Autodesk Inventor part; units mm, degrees
ref_plane "YZ Plane" through (0, 0, 0) normal (1, 0, 0) x (0, 1, 0)
ref_plane "XZ Plane" through (0, 0, 0) normal (0, 1, 0) x (-1, 0, 0)
ref_plane "XY Plane" through (0, 0, 0) normal (0, 0, 1) x (1, 0, 0)
sketch "Sketch1" plane through (0, 0, 0) normal (0, 0, 1) x (1, 0, 0)
  circle A0 centre (0, 0) radius 374.904
  dimension "d0" = 749.808
extrude "Extrusion1" add sketch "Sketch1" along normal blind 25.4
sketch "Sketch2" plane through (0, 0, 0) normal (0, 0, 1) x (1, 0, 0)
  circle A0 centre (0, 0) radius 355.854
  dimension "d3" = 711.708
extrude "Extrusion2" add sketch "Sketch2" along normal blind 50
sketch "Sketch3" plane through (0, 0, 0) normal (0, 0, 1) x (1, 0, 0)
  circle A0 centre (0, 0) radius 349.25
  dimension "d6" = 698.5
extrude "Extrusion3" add sketch "Sketch3" along normal blind 1330.7314
sketch "Sketch4" plane through (0, 0, 1330.7314) normal (0, 0, 1) x (1, 0, 0)
  circle A0 centre (-6.35, 0) radius 317.5
  point P0 (0, 0)
  dimension "d9" = 635
  dimension "d21" = 6.35
extrude "Extrusion4" cut sketch "Sketch4" against normal through all
chamfer "Chamfer1" distance 0.7937 angle 45 1 edges at (-374.904, 0, 25.4)
fillet "Fillet1" radius 0.7937 1 edges at (-355.854, 0, 25.4)
fillet "Fillet2" radius 0.7937 1 edges at (-349.25, 0, 50)
sketch "Sketch5" plane through (0, 0, 0) normal (0, 1, 0) x (-1, 0, 0)
  line L0 (-311.15, 1330.7314) -> (323.85, 1330.7314)
  line L1 (-311.15, 1330.7314) -> (323.85, 797.9031)
  line L2 (323.85, 797.9031) -> (349.25, 797.9031)
  line L3 (349.25, 797.9031) -> (349.25, 1330.7314)
  line L4 (349.25, 1330.7314) -> (323.85, 1330.7314)
  line L5 (349.25, 50.7937) -> (349.25, 1330.7314) construction
  point P0 (0, 0)
  dimension "d18" = 40
extrude "Extrusion5" cut sketch "Sketch5" along normal through all both and the other way through all
properties part number "A1-19010-200-02 HCWI nozzle insert" material "Iron, Cast"
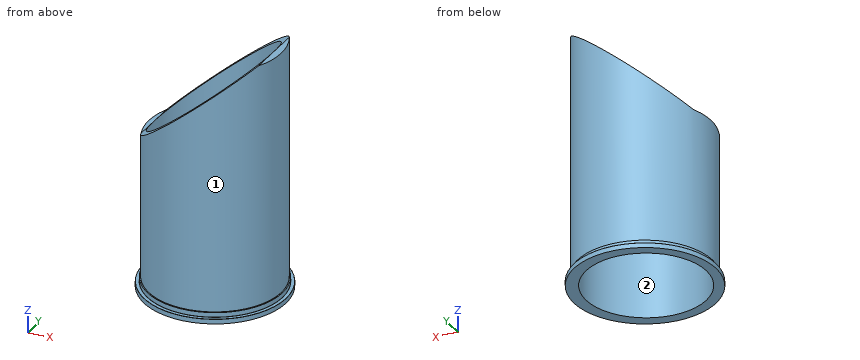
For this review, take the finished solid that the model builds, in its own axes (mm). Face numbers are marked on the shaded views. Give positions to 0.01 mm unless a question says otherwise; leave off trailing zeros. Loops run counter-clockwise (first coordinate to the right, second up) from the corner with the lowest first, then second, coordinate; pieces in that order, holes last. Notation, with made-up numbers: M 60.25,-5 L 83.25,-5 A20 cw 83.25,13 Z; hole C 64,54 d7. An arc over 180 degrees is marked long. Answer as a JSON object with one key per item and string values. Group by question number.
Q1. Add section A-A on z = 229.5. Give the boundary of the cut face in (x, y), and give its area (3 significant figures).
Q2. Add section B-B on x = 0. Give the boundary of the cut face in (y, z).
Q3. For probe 1 along Y at (x, z) = (-6.35, 566.5); probe 2 along X at (y, z) = (0, 477); probe 3 along X at (y, z) = (0, 805), list the stretches that pass through material, from the lowest coordinate up. Write a range as [from, to].
Q4. Mouldability with a two-part tool opening along X and no side actions: class the marked faces 1 and 2 as +X half, -X half, draft (parallel to the pull), parting line (faces both ways), or undercut.
Q5. Add section C-C on z = 912. Give the boundary of the cut face in (x, y), and give its area (3 significant figures).
Q6. Insertion check: P1, Ø1, axis at y = -79, z = 894, coming from the +X side; P2, Ø8, axis at y = -96.5, z = 751.5, coming from the -X side; P3, Ø20.5, axis at x = -334, y = 59.5, coming from the +Z side. Each pin has a flat end and moves straight along its axis. Give the tip position at first contact, or say it passes through.
Checked values:
{
 "1": {"outline": "C 0,0 d698.5; hole C -6.35,0 d635", "area": "66,500 mm²"},
 "2": {"outline": "M -374.9,0 L -317.44,0 L -317.44,1069.65 L -349.25,1069.65 L -349.25,50.79 A0.79 cw -350.04,50 L -355.85,50 L -355.85,26.19 A0.79 cw -356.65,25.4 L -374.11,25.4 L -374.9,24.61 Z; M 317.44,0 L 374.9,0 L 374.9,24.61 L 374.11,25.4 L 356.65,25.4 A0.79 cw 355.85,26.19 L 355.85,50 L 350.04,50 A0.79 cw 349.25,50.79 L 349.25,1069.65 L 317.44,1069.65 Z"},
 "3": {"probe 1": "[-349.19, -317.5], [317.5, 349.19]", "probe 2": "[-349.25, -323.85], [311.15, 349.25]", "probe 3": "[311.15, 349.25]"},
 "4": {"face 1": "parting line", "face 2": "undercut"},
 "5": {"outline": "M -187.87,-294.41 A349.25 ccw long -187.87,294.41 L -187.87,260.49 A317.5 cw long -187.87,-260.49 Z", "area": "49,200 mm²"},
 "6": {"P1": "x = 340.31", "P2": "x = -336.78", "P3": "z = 797.99"}
}
